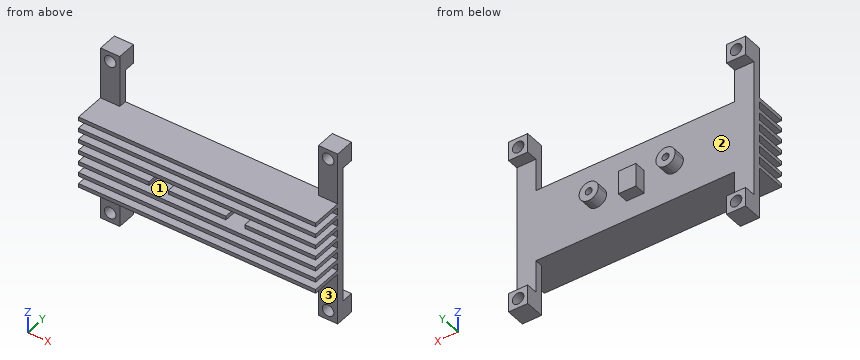
```python
from build123d import *

# Parameters (mm, degrees)
F1_DEPTH = 10
F2_W     = 5
F2_H     = 13.5
F2_W_2   = 61.75
F2_H_2   = 2
F4_DEPTH = 8
F5_W     = 5
F5_H     = 5
F5_R     = 1.5
F5_R_2   = 0.9
F5_W_2   = 4.6
F5_H_2   = 6.1
F7_DEPTH = 5
F8_DEPTH = 8.001
F9_DEPTH = 5.001


# Not quite as in the source:
# - a feature names something its author has since deleted; it is built from what else it names


with BuildPart() as f1:
    # F0 (on Front) → F1 (new body)
    with BuildSketch(Plane.XZ):
        Polygon((-25.875, 23), (-30.875, 23), (-30.875, -23), (-25.875, -23), (-25.875, -9.5), (0, -9.5), (25.875, -9.5), (25.875, -23), (30.875, -23), (30.875, 23), (25.875, 23), (25.875, 9.5), (0, 9.5), (-25.875, 9.5), align=None)
    extrude(amount=F1_DEPTH)

    # F2 (on face) → F4 (cut, through all)
    with BuildSketch(Plane.XZ.offset(10)):
        with Locations((-28.375, 16.25)):
            Rectangle(F2_W, F2_H)
        with Locations((0, 7.5)):
            Rectangle(F2_W_2, F2_H_2)
        with Locations((0, 4.5)):
            Rectangle(F2_W_2, F2_H_2)
        with Locations((0, 1.5)):
            Rectangle(F2_W_2, F2_H_2)
        with Locations((0, -1.5)):
            Rectangle(F2_W_2, F2_H_2)
        with Locations((0, -4.5)):
            Rectangle(F2_W_2, F2_H_2)
        with Locations((0, -7.5)):
            Rectangle(F2_W_2, F2_H_2)
        with Locations((-28.375, -16.25)):
            Rectangle(F2_W, F2_H)
        with Locations((28.375, 16.25)):
            Rectangle(F2_W, F2_H)
        with Locations((28.375, -16.25)):
            Rectangle(F2_W, F2_H)
    extrude(amount=-F4_DEPTH, mode=Mode.SUBTRACT)

    # F5 (on offset) → F7 (join, through all)
    with BuildSketch(Plane.XZ.offset(2)):
        with Locations((-28.375, 20.5)):
            Rectangle(F5_W, F5_H)
        with Locations((-28.375, 20.5)):
            Circle(F5_R, mode=Mode.SUBTRACT)
        with Locations((28.375, 20.5)):
            Rectangle(F5_W, F5_H)
        with Locations((28.375, 20.5)):
            Circle(F5_R, mode=Mode.SUBTRACT)
        with Locations((28.375, -20.5)):
            Rectangle(F5_W, F5_H)
        with Locations((28.375, -20.5)):
            Circle(F5_R, mode=Mode.SUBTRACT)
        with Locations((-28.375, -20.5)):
            Rectangle(F5_W, F5_H)
        with Locations((-28.375, -20.5)):
            Circle(F5_R, mode=Mode.SUBTRACT)
        with BuildLine():
            ThreePointArc((10, 2.5), (8.232233047, 1.767766953), (7.5, 0))
            ThreePointArc((7.5, 0), (8.232233047, -1.767766953), (10, -2.5))
            ThreePointArc((10, -2.5), (11.767766953, -1.767766953), (12.5, 0))
            ThreePointArc((12.5, 0), (11.767766953, 1.767766953), (10, 2.5))
        make_face()
        with Locations((10, 0)):
            Circle(F5_R_2, mode=Mode.SUBTRACT)
        with BuildLine():
            ThreePointArc((-10, -2.5), (-8.232233047, -1.767766953), (-7.5, 0))
            ThreePointArc((-7.5, 0), (-8.232233047, 1.767766953), (-10, 2.5))
            ThreePointArc((-10, 2.5), (-11.767766953, 1.767766953), (-12.5, 0))
            ThreePointArc((-12.5, 0), (-11.767766953, -1.767766953), (-10, -2.5))
        make_face()
        with Locations((-10, 0)):
            Circle(F5_R_2, mode=Mode.SUBTRACT)
        with Locations((0, -1.25)):
            Rectangle(F5_W_2, F5_H_2)
    extrude(amount=-F7_DEPTH)

    # F5 (on offset) → F8 (cut, through all)
    with BuildSketch(Plane.XZ.offset(2)):
        with BuildLine():
            ThreePointArc((-10, 2.5), (-8.232233047, 1.767766953), (-7.5, 0))
            Line((-7.5, 0), (-7.5, 2.5))
            Line((-7.5, 2.5), (-10, 2.5))
        make_face()
        with BuildLine():
            ThreePointArc((-12.5, 0), (-11.767766953, 1.767766953), (-10, 2.5))
            Line((-10, 2.5), (-12.5, 2.5))
            Line((-12.5, 2.5), (-12.5, 0))
        make_face()
        with BuildLine():
            Line((-12.5, -2.5), (-10, -2.5))
            ThreePointArc((-10, -2.5), (-11.767766953, -1.767766953), (-12.5, 0))
            Line((-12.5, 0), (-12.5, -2.5))
        make_face()
        with BuildLine():
            Line((-7.5, -2.5), (-7.5, 0))
            ThreePointArc((-7.5, 0), (-8.232233047, -1.767766953), (-10, -2.5))
            Line((-10, -2.5), (-7.5, -2.5))
        make_face()
        with BuildLine():
            ThreePointArc((-10, -2.5), (-8.232233047, -1.767766953), (-7.5, 0))
            ThreePointArc((-7.5, 0), (-8.232233047, 1.767766953), (-10, 2.5))
            ThreePointArc((-10, 2.5), (-11.767766953, 1.767766953), (-12.5, 0))
            ThreePointArc((-12.5, 0), (-11.767766953, -1.767766953), (-10, -2.5))
        make_face()
        with Locations((-10, 0)):
            Circle(F5_R_2, mode=Mode.SUBTRACT)
        with Locations((-10, 0)):
            Circle(F5_R_2)
        with BuildLine():
            Line((10, 2.5), (7.5, 2.5))
            Line((7.5, 2.5), (7.5, 0))
            ThreePointArc((7.5, 0), (8.232233047, 1.767766953), (10, 2.5))
        make_face()
        with BuildLine():
            ThreePointArc((10, -2.5), (8.232233047, -1.767766953), (7.5, 0))
            Line((7.5, 0), (7.5, -2.5))
            Line((7.5, -2.5), (10, -2.5))
        make_face()
        with BuildLine():
            ThreePointArc((10, 2.5), (8.232233047, 1.767766953), (7.5, 0))
            ThreePointArc((7.5, 0), (8.232233047, -1.767766953), (10, -2.5))
            ThreePointArc((10, -2.5), (11.767766953, -1.767766953), (12.5, 0))
            ThreePointArc((12.5, 0), (11.767766953, 1.767766953), (10, 2.5))
        make_face()
        with Locations((10, 0)):
            Circle(F5_R_2, mode=Mode.SUBTRACT)
        with Locations((10, 0)):
            Circle(F5_R_2)
    extrude(amount=F8_DEPTH, mode=Mode.SUBTRACT)

    # F5 (on offset) → F9 (cut, through all)
    with BuildSketch(Plane.XZ.offset(2)):
        with Locations((28.375, 20.5)):
            Circle(F5_R)
        with Locations((10, 0)):
            Circle(F5_R_2)
        with Locations((-10, 0)):
            Circle(F5_R_2)
        with Locations((28.375, -20.5)):
            Circle(F5_R)
        with Locations((-28.375, -20.5)):
            Circle(F5_R)
        with Locations((-28.375, 20.5)):
            Circle(F5_R)
    extrude(amount=-F9_DEPTH, mode=Mode.SUBTRACT)


solid = f1.part
```
Could you check a few things on this model? Use its own coordinates, in mm. Face numbers are marked on the shaded views. A direction names the side the tool comes from. Give positions to 0.01 mm unless a question says otherwise; leave off trailing zeros. Order: outer loops, then holes, each group sorted by start corner. A loop starts at its lowest first (then second) coordinate and runs counter-clockwise, first axis right, second up.
Q1. Suppose I cut it at B-B, the plane x = 21. Write out the boundary of the cut face in (y, z), and give its area (3 significant figures).
Q2. Suppose I cut it at A-A, the plane z = -17. Write out the boundary of the cut face in (x, y) (3 decimals), and give its area (3 significant figures).
Q3. For the marked faces 1, 2 and 3, which set-ups out of +Z, -Z, +X, -X, +Y, -Y let a thin tool reach every point of the face, with its end or its side?
Q4. Suppose I cut it at D-D, the plane y = -8.5. Count the separate pieces of the cut face and the enclosed holes in it, and give its area (3 significant figures).
Q5. If I drill on line 1 along Z through (x, y) = (12, -6); line 2 along X through (y, z) = (2.25, -0.5); line 3 along Y through (x, z) = (-7.5, 6), over which ranges is the centre line in solid material (lowest first)?
Q6. Suppose I cut it at C-C, the plane z = 20.5. Write out the boundary of the cut face in (x, y) (3 decimals).
Q7. I'm going to push flat-ended pins straight in: P1, Ø1.5, axis at x = 29, z = 19, coming from the -Y side; P2, Ø2.5, axis at x = -28.375, z = 20.5, coming from the -Y side; P3, Ø6, axis at x = -18.5, y = -1.5, coming from the -Z side; P4, Ø0.9, axis at x = 0, y = 2, coming from the +Z side. Where does each tip first touch, or does it pass through?
Solution:
1. outline: (-10, -9.5) - (0, -9.5) - (0, 9.5) - (-10, 9.5) - (-10, 8.5) - (-2, 8.5) - (-2, 6.5) - (-10, 6.5) - (-10, 5.5) - (-2, 5.5) - (-2, 3.5) - (-10, 3.5) - (-10, 2.5) - (-2, 2.5) - (-2, 0.5) - (-10, 0.5) - (-10, -0.5) - (-2, -0.5) - (-2, -2.5) - (-10, -2.5) - (-10, -3.5) - (-2, -3.5) - (-2, -5.5) - (-10, -5.5) - (-10, -6.5) - (-2, -6.5) - (-2, -8.5) - (-10, -8.5) - close
1. area: 94.0 mm2
2. outline: (-30.875, -2) - (-25.875, -2) - (-25.875, 0) - (-30.875, 0) - close; (25.875, -2) - (30.875, -2) - (30.875, 0) - (25.875, 0) - close
2. area: 20.0 mm2
3. face 1: +X, -X, -Y
3. face 2: +Y
3. face 3: -Z, +X, -X, -Y
4. separate pieces: 9
4. enclosed holes: 0
4. area: 422 mm2
5. line 1: z = -9.5 to -8.5, -6.5 to -5.5, -3.5 to -2.5, 2.5 to 3.5, 5.5 to 6.5, 8.5 to 9.5
5. line 2: x = -12.45 to -10.75, -9.25 to -7.55, -2.3 to 2.3, 7.55 to 9.25, 10.75 to 12.45
5. line 3: y = -10 to 0
6. outline: (-30.875, -2) - (-29.875, -2) - (-29.875, 3) - (-30.875, 3) - close; (-26.875, -2) - (-25.875, -2) - (-25.875, 3) - (-26.875, 3) - close; (25.875, -2) - (26.875, -2) - (26.875, 3) - (25.875, 3) - close; (29.875, -2) - (30.875, -2) - (30.875, 3) - (29.875, 3) - close
7. P1: stops at y = -2
7. P2: passes through
7. P3: stops at z = -9.5
7. P4: stops at z = 1.8
